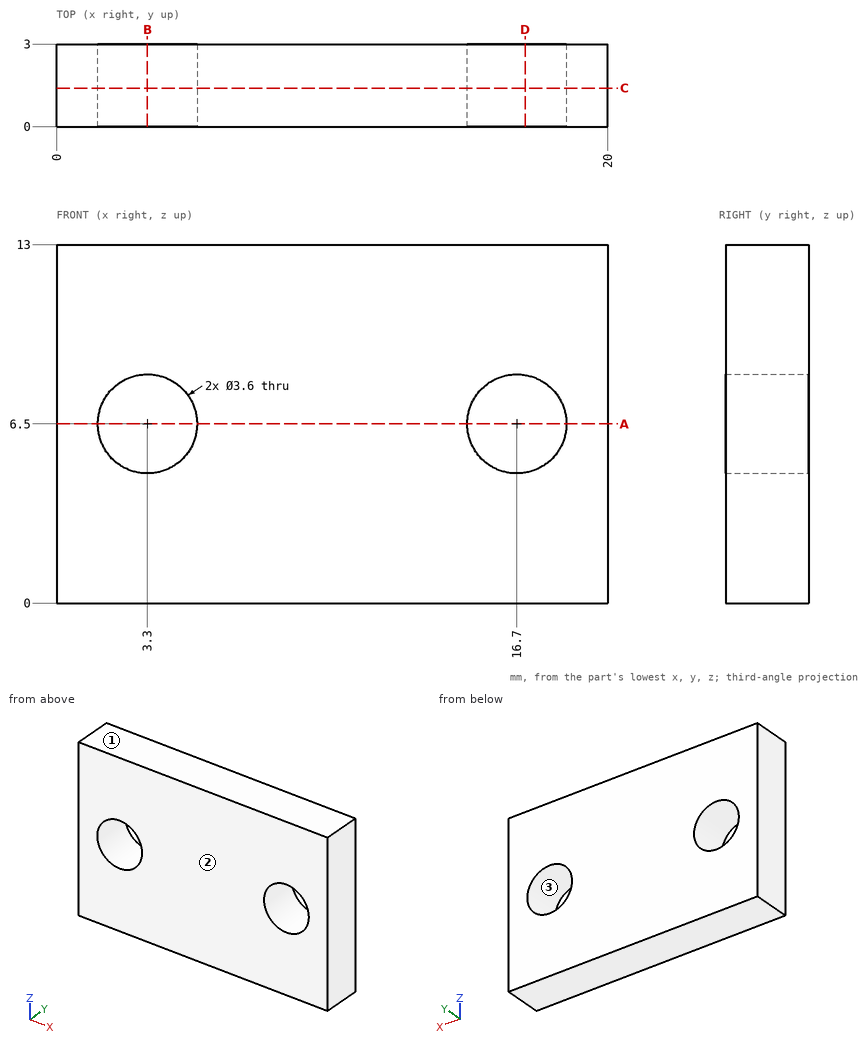
Here's the drawing with two shaded views (mm, measured from the low corner). I have some questions. Coordinates: 2 decimals unless noted, no trailing zeros. Write each loop counter-clockwise with the first axis right and the second up, starting at its lowest first coordinate (ties: lowest second). Pieces come first, ordered by that corner, then holes. Notation, with made-up numbers: (-22, 20.25) - (-10, 20.25) arc R21 ccw to (-10, 40.25) - close; hole circle Ø2 at (12.25, 24.25). An arc over 180 degrees is marked (long way). Return JSON: item names as keys, results as strings.
Q1. If we section it at D-D (x = 17): Please give me the cut outline in (y, z).
Computed values:
{"outline": "(0, 0) - (3, 0) - (3, 4.73) - (0, 4.73) - close; (0, 8.27) - (3, 8.27) - (3, 13) - (0, 13) - close"}
Q2. If we section it at C-C (y = 1.4): Please give me the cut outline in (x, z).
Computed values:
{"outline": "(0, 0) - (20, 0) - (20, 13) - (0, 13) - close; hole circle Ø3.6 at (3.3, 6.5); hole circle Ø3.6 at (16.7, 6.5)"}
Q3. If we section it at B-B (x = 3.3): Please give me the cut outline in (y, z), then the cut area to 3 significant figures.
Computed values:
{"outline": "(0, 0) - (3, 0) - (3, 4.7) - (0, 4.7) - close; (0, 8.3) - (3, 8.3) - (3, 13) - (0, 13) - close", "area": "28.2 mm2"}
Q4. Please list where these lines run through material, in increasing order: L1, parallel to X at y = 0.9, z = 6.5; L2, parallel to Z at x = 16.7, y = 0.65; L3, parallel to X at y = 2.95, z = 8. Write a range as from..to.
Computed values:
{"L1": "x = 0..1.5, 5.1..14.9, 18.5..20", "L2": "z = 0..4.7, 8.3..13", "L3": "x = 0..2.31, 4.29..15.71, 17.69..20"}
Q5. Thinking about a two-plate mould opening in Z: for the marked faces 1, 2 and 3, which applies, +Z half, -Z half, draft (parallel to the pull), parting line (faces both ways), or undercut?
Computed values:
{"face 1": "+Z half", "face 2": "draft", "face 3": "undercut"}
Q6. If we section it at A-A (z = 6.5): Please give me the cut outline in (x, y).
Computed values:
{"outline": "(0, 0) - (1.5, 0) - (1.5, 3) - (0, 3) - close; (5.1, 0) - (14.9, 0) - (14.9, 3) - (5.1, 3) - close; (18.5, 0) - (20, 0) - (20, 3) - (18.5, 3) - close"}
